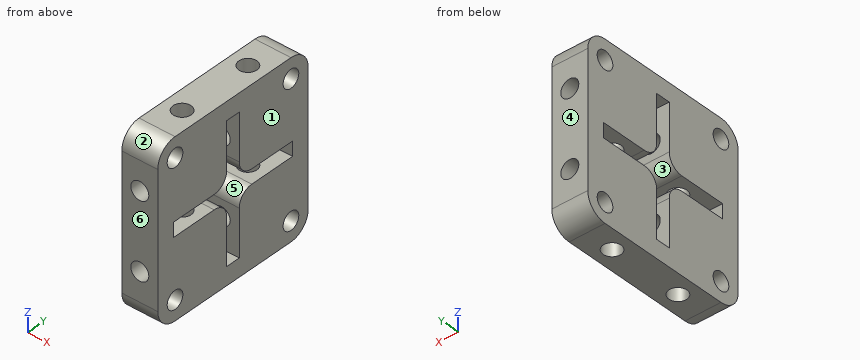
Autodesk Inventor part; units mm, degrees
ref_plane "YZ Plane" through (0, 0, 0) normal (1, 0, 0) x (0, 1, 0)
ref_plane "XZ Plane" through (0, 0, 0) normal (0, 1, 0) x (-1, 0, 0)
ref_plane "XY Plane" through (0, 0, 0) normal (0, 0, 1) x (1, 0, 0)
sketch "Sketch1" plane through (0, 0, 0) normal (1, 0, 0) x (0, 1, 0)
  circle A0 centre (0, 0) radius 2.8284
  line L0 (0, 0) -> (-2.8284, 0)
  line L1 (-2.8284, 0) -> (-2.8284, -2.8284)
  line L2 (-2.8284, -2.8284) -> (0, -2.8284)
  line L3 (0, -2.8284) -> (0, 0)
  line L4 (0, 0) -> (-2.8284, -2.8284)
  line L5 (2, 2) -> (-2, 2)
  line L6 (-2, 2) -> (-2, -2)
  line L7 (-2, -2) -> (2, -2)
  line L8 (2, -2) -> (2, 2)
  line L9 (2, 2) -> (-2, -2) construction
  line L10 (-2, 2) -> (2, -2) construction
  line L11 (2, 2) -> (-2, 2)
  line L12 (-2, 2) -> (-2, 4)
  line L13 (-2, 4) -> (2, 4)
  line L14 (2, 4) -> (2, 2)
  line L15 (0, 4) -> (0, 19)
  line L16 (-2, 2) -> (-4, 2)
  line L17 (-4, 2) -> (-4, -2)
  line L18 (-4, -2) -> (-2, -2)
  line L19 (-4, 0) -> (-19, 0)
  line L20 (19, -19) -> (19, 19)
  line L21 (19, 19) -> (-19, 19)
  line L22 (-19, 19) -> (-19, -19)
  line L23 (-19, -19) -> (19, -19)
  line L24 (19, -19) -> (-19, 19) construction
  line L25 (19, 19) -> (-19, -19) construction
  line L26 (0, 19) -> (0, 24)
  line L27 (-19, 0) -> (-24, 0)
  line L28 (24, -24) -> (24, 24)
  line L29 (24, 24) -> (-24, 24)
  line L30 (-24, 24) -> (-24, -24)
  line L31 (-24, -24) -> (24, -24)
  line L32 (24, -24) -> (-24, 24) construction
  line L33 (24, 24) -> (-24, -24) construction
  line L34 (-2, 2) -> (-19, 2)
  line L35 (-19, -2) -> (-2, -2)
  line L36 (-2, -2) -> (-2, 2)
  line L37 (-2, -2) -> (-19, -2)
  line L38 (-19, -2) -> (-19, -19)
  line L39 (-19, -19) -> (-2, -19)
  line L40 (-2, -19) -> (-2, -2)
  line L41 (2, -2) -> (19, -2)
  line L42 (19, -2) -> (19, -19)
  line L43 (19, -19) -> (2, -19)
  line L44 (2, -19) -> (2, -2)
  line L45 (2, 2) -> (19, 2)
  line L46 (19, 2) -> (19, 19)
  line L47 (19, 19) -> (2, 19)
  line L48 (2, 19) -> (2, 2)
  line L49 (-2, 2) -> (-19, 2)
  line L50 (-19, 2) -> (-19, 19)
  line L51 (-19, 19) -> (-2, 19)
  line L52 (-2, 19) -> (-2, 2)
  point P0 (-2, 19)
  point P1 (2, 4)
  point P2 (2, -19)
  point P3 (-2, -19)
  dimension "d0" = 4
  dimension "d1" = 2
  dimension "d5" = 15
  dimension "d6" = 2
  dimension "d7" = 15
  dimension "d8" = 2
  dimension "d9" = 0
  dimension "d10" = 5
  dimension "d11" = 5
  dimension "d12" = 15
  dimension "d13" = 22.6716
  dimension "d14" = 20
  dimension "d15" = 29.7321
extrude "Extrusion1" add sketch "Sketch1" along normal blind 10 contours L14 L48 L21 L20 L45 | L41 L20 L23 L44 | L16 L34 L22 L21 L52 L12 | L20 L21 L26 L29 L28 L31 L30 L27 L22 L23 | L40 L2 L4 | L4 L1 L18 | L40 L23 L22 L35 L18 L1 L2 | L21 L22 L27 L30 L29 L26
sketch "Sketch2" plane through (0, 24, 24) normal (0, 1, 0) x (1, 0, 0)
  line L0 (10, 0) -> (0, 0)
  line L1 (0, 0) -> (0, 48)
  line L2 (0, 48) -> (10, 48)
  line L3 (10, 48) -> (10, 0)
  line L4 (0, 48) -> (10, 48)
  line L5 (0, 48) -> (0, 34.5)
  line L6 (0, 34.5) -> (5, 34.5)
  circle A0 centre (5, 34.5) radius 2.5
  line L7 (0, 0) -> (0, 13.5)
  line L8 (0, 22) -> (0, 5)
  line L9 (0, 13.5) -> (5, 13.5)
  circle A1 centre (5, 13.5) radius 2.5
  point P0 (0, 24)
  dimension "d18" = 13.5
  dimension "d19" = 5
  dimension "d20" = 5
  dimension "d21" = 13.5
  dimension "d22" = 5
  dimension "d23" = 5
extrude "Extrusion2" cut sketch "Sketch2" against normal through all contours A0 | A1
sketch "Sketch3" plane through (0, -24, -24) normal (0, 0, -1) x (-1, 0, 0)
  line L0 (0, 0) -> (-10, 0)
  line L1 (0, 0) -> (0, 13.5)
  line L2 (0, 22) -> (0, 5)
  line L3 (0, 48) -> (-10, 48)
  line L4 (0, 48) -> (0, 34.5)
  line L5 (0, 0) -> (0, 48)
  line L6 (0, 34.5) -> (-5, 34.5)
  line L7 (0, 13.5) -> (-5, 13.5)
  circle A0 centre (-5, 13.5) radius 2.5
  circle A1 centre (-5, 34.5) radius 2.5
  point P0 (0, 24)
  dimension "d26" = 13.5
  dimension "d27" = 13.5
  dimension "d28" = 5
  dimension "d29" = 5
  dimension "d30" = 5
  dimension "d31" = 5
extrude "Extrusion3" cut sketch "Sketch3" against normal through all
fillet "Fillet1" radius 4 4 edges at (5, -2, 2) (5, 2, 2) (5, 2, -2) (5, -2, -2)
sketch "Sketch4" plane through (10, 0, 0) normal (1, 0, 0) x (0, 0, -1)
  line L0 (24, 24) -> (-24, 24)
  line L1 (24, 24) -> (18.5, 24)
  line L2 (18.5, 24) -> (18.5, 18.5)
  line L3 (18.5, 18.5) -> (24, 18.5)
  line L4 (24, 18.5) -> (24, 24)
  circle A0 centre (18.5, 18.5) radius 2.5
  circle A1 centre (18.5, 18.5) radius 5.5
  circle A2 centre (-18.5, 18.5) radius 5.5
  circle A3 centre (-18.5, 18.5) radius 2.5
  line L5 (-18.5, 24) -> (-24, 24)
  line L6 (-24, 24) -> (-24, 18.5)
  circle A4 centre (-18.5, -18.5) radius 5.5
  circle A5 centre (-18.5, -18.5) radius 2.5
  line L7 (-24, -18.5) -> (-24, -24)
  line L8 (-24, -24) -> (-18.5, -24)
  circle A6 centre (18.5, -18.5) radius 5.5
  circle A7 centre (18.5, -18.5) radius 2.5
  line L9 (18.5, -24) -> (24, -24)
  line L10 (24, -24) -> (24, -18.5)
  point P0 (0, 0)
  point P1 (-18.5, 24)
  dimension "d35" = 5.5
  dimension "d36" = 5.5
  dimension "d37" = 5
  dimension "d40" = 360
extrude "Extrusion4" cut sketch "Sketch4" against normal through all contours L4 A1 L0 | A2 L6 L0 | A0 L3 L2 | L2 L3 A0 | A3 | A4 L8 L7 | A5 | L10 L9 A6 | A7
properties part number "guidance_block"
Could you check a few things on this model? Use its own coordinates, in mm. Face numbers are marked on the shaded views. A direction names the side the tool comes from. Give positions to 0.01 mm unless a question says otherwise; leave off trailing zeros. Order: outer loops, then holes, each group sorted by start corner. A loop starts at its lowest first (then second) coordinate and runs counter-clockwise, first axis right, second up. Notation, with made-up numbers: (73, 36.25) -> (94, 36.25) arc R7 ccw to (94, 44.25) -> close; hole circle Ø3 at (67.5, 39). An arc over 180 degrees is marked (long way). Answer in a Markdown table with one row per item. Add a question column.
Item 1: Imagine slicing it at B-B (z = -0.5). List the corners of the cut face in (x, y) for me.
Item 2: For the marked faces 5 and 6, which set-ups out of +Z, -Z, +X, -X, +Y, -Y let a thin tool reach every point of the face, with its end or its side?
Item 3: We'd pull the mould along Y, two halves only. Please class the marked faces 1, 2, 3 and 4: pulls with the +Y half, pulls with the -Y half, needs draft (parallel to the pull), parting line crosses it, or undercut.
Item 4: Please list where these lines run through material, in increasing order: probe 1 along Z at (x, y) = (5, -7.5); probe 2 along X at (y, z) = (-10.5, -6.75); probe 3 along Z at (x, y) = (7.25, -8).
Item 5: I'm going to push a flat-ended pin straight in: P1, Ø3, axis at x = 5, z = -10.5, coming from the -Y side (1 decimal). Where does the tip first touch, or does it pass through?
Item 6: Imagine slicing it at A-A (y = -9). List the corners of the cut face in (x, z) for me.
Result:
| question | item | result |
|---|---|---|
| 1 | outline | (0, -24) -> (10, -24) -> (10, -19) -> (0, -19) -> close; (0, 19) -> (10, 19) -> (10, 24) -> (0, 24) -> close |
| 2 | face 5 | +X, -X |
| 2 | face 6 | +Z, -Z, +X, -X, -Y |
| 3 | face 1 | needs draft |
| 3 | face 2 | pulls with the -Y half |
| 3 | face 3 | undercut |
| 3 | face 4 | pulls with the +Y half |
| 4 | probe 1 | -24 to -13, -8 to -2, 2 to 8, 13 to 24 |
| 4 | probe 2 | 0 to 2.5, 7.5 to 10 |
| 4 | probe 3 | -24 to -11.59, -9.41 to -2, 2 to 9.41, 11.59 to 24 |
| 5 | P1 | through |
| 6 | outline | (0, -24) -> (3, -24) -> (3, -12) arc R2.5 cw to (3, -9) -> (3, -2) -> (0, -2) -> close; (0, 2) -> (3, 2) -> (3, 9) arc R2.5 cw to (3, 12) -> (3, 24) -> (0, 24) -> close; (7, -24) -> (10, -24) -> (10, -2) -> (7, -2) -> (7, -9) arc R2.5 cw to (7, -12) -> close; (7, 2) -> (10, 2) -> (10, 24) -> (7, 24) -> (7, 12) arc R2.5 cw to (7, 9) -> close |
